from build123d import *

# Parameters (mm, degrees)
BASE_FLANGE3_DEPTH       = 425
SKETCH21_W               = 50
SKETCH21_H               = 5
BOSS_EXTRUDE2_DEPTH      = 50
CHAMFER1_SIZE            = 5
SKETCH26_R               = 9
CUT_EXTRUDE1_DEPTH       = 50
CHAMFER1_OF_MIRROR1_SIZE = 5


# Sheet-metal steps are written as plain solids
with BuildPart() as part:
    # Sketch1 → Base-Flange3 (new, symmetric)
    with BuildSketch(Plane.XY):
        with BuildLine():
            Line((63.8, 0), (63.8, 27.625))
            ThreePointArc((63.8, 27.625), (65.901508845, 32.698491155), (70.975, 34.8))
            Line((70.975, 34.8), (132.825, 34.8))
            ThreePointArc((132.825, 34.8), (137.898491155, 32.698491155), (140, 27.625))
            Line((140, 27.625), (140, 0))
            Line((140, 0), (136.825, 0))
            Line((136.825, 0), (136.825, 27.625))
            ThreePointArc((136.825, 27.625), (135.653427125, 30.453427125), (132.825, 31.625))
            Line((132.825, 31.625), (70.975, 31.625))
            ThreePointArc((70.975, 31.625), (68.146572875, 30.453427125), (66.975, 27.625))
            Line((66.975, 27.625), (66.975, 0))
            Line((66.975, 0), (63.8, 0))
        make_face()
    extrude(amount=BASE_FLANGE3_DEPTH, both=True)

    # Sketch21 → Boss-Extrude2 (add)
    with BuildSketch(Plane(origin=(140, 0, 0), x_dir=(0, 0, -1), z_dir=(1, 0, 0))):
        with Locations((-225, 2.5)):
            Rectangle(SKETCH21_W, SKETCH21_H)
    boss_extrude2 = extrude(amount=BOSS_EXTRUDE2_DEPTH)

    # Chamfer1
    chamfer1_edges = [part.edges().sort_by_distance(p)[0] for p in [
        (190, 2.5, 250),
        (190, 2.5, 200),
    ]]
    chamfer(chamfer1_edges, length=CHAMFER1_SIZE)

    # Sketch26 → Cut-Extrude1 (cut)
    with BuildSketch(Plane(origin=(0, 5, 0), x_dir=(1, 0, 0), z_dir=(0, 1, 0))):
        with Locations(Location((165, -225, 0), (0, 0, 270))):
            Circle(SKETCH26_R)
    cut_extrude1 = extrude(amount=-CUT_EXTRUDE1_DEPTH, mode=Mode.SUBTRACT)

    # Mirror1: Boss-Extrude2, Cut-Extrude1 across plane
    add(boss_extrude2.mirror(Plane.XY))
    add(cut_extrude1.mirror(Plane.XY), mode=Mode.SUBTRACT)

    # Chamfer1 of Mirror1
    chamfer1_of_mirror1_edges = [part.edges().sort_by_distance(p)[0] for p in [
        (190, 2.5, -250),
        (190, 2.5, -200),
    ]]
    chamfer(chamfer1_of_mirror1_edges, length=CHAMFER1_OF_MIRROR1_SIZE)


solid = part.part
Work out the finished part from the listing and answer in its coordinate system (mm). A direction names the side the tool comes from. Give positions to 0.01 mm unless a question says otherwise; leave off trailing zeros. Order: outer loops, then holes, each group sorted by start corner. A loop starts at its lowest first (then second) coordinate and runs counter-clockwise, first axis right, second up. Notation, with made-up numbers: (66.25, 66) - (78.25, 66) arc R19 ccw to (78.25, 84) - close; hole circle Ø8 at (67, 29.25). An arc over 180 degrees is marked (long way). Answer as CSV lines item,"result". Start each with the question number.
Q1. Find the intervals of material crossed by L1, parallel to X at y = 2.05, z = 225 (3 decimals); L2, parallel to X at y = 13, z = -217 (3 decimals); L3, parallel to Y at x = 83.5, z = 259.5 (3 decimals), in increasing order. Write a range as [from, to].
Q2. The part is cut by section B-B (z = -225). Write down the section's boundary in (x, y) (3 decimals).
Q3. The part is cut by section A-A (y = 21). Write down the section's boundary in (x, z) (3 decimals).
Q4. The part is cut by section D-D (z = 364.5). Write down the section's boundary in (x, y) (3 decimals), then the cut area to 3 significant figures.
Q5. For faces 4 (the face through (66.975, 14, 6)), 5 (the face through (165, 5, -214)), 6 (the face through (138, 0, -61)), determine the directions among +Z, -Z, +X, -X, +Y, -Y from which every point of the face is accessible in a straight line to the end or side of a thin tool.
Q6. Given pin 1 Ø18.5 at (x, z) = (117.5, 83.5) entering from -Y (3 decimals); pin 2 Ø14 at (y, z) = (20.5, -30.5) entering from +X; pin 3 Ø8 at (x, y) = (169, 7.5) entering from +Z, each flat-ended and moving along its own axis, determine where each tip first touches the part or whether it passes through.
Q7. The part is cut by section C-C (x = 165). Write down the section's boundary in (y, z).
Q8. The mould has two halves that part along Z. Classify faces 1 (the face through (102, 32, 425)), 2 (the face through (171.083, 2.535, -218.367)), 3 (the face through (102, 31.625, 6)): +Z half, -Z half, draft (parallel to the pull), parting line (faces both ways), or undercut.
Check result:
1,L1,"x = [63.8, 66.975], [136.825, 156], [174, 190]"
1,L2,"x = [63.8, 66.975], [136.825, 140]"
1,L3,"y = [31.625, 34.8]"
2,outline,"(63.8, 0) - (66.975, 0) - (66.975, 27.625) arc R4 cw to (70.975, 31.625) - (132.825, 31.625) arc R4 cw to (136.825, 27.625) - (136.825, 0) - (156, 0) - (156, 5) - (140, 5) - (140, 27.625) arc R7.175 ccw to (132.825, 34.8) - (70.975, 34.8) arc R7.175 ccw to (63.8, 27.625) - close; (174, 0) - (190, 0) - (190, 5) - (174, 5) - close"
3,outline,"(63.8, -425) - (66.975, -425) - (66.975, 425) - (63.8, 425) - close; (136.825, -425) - (140, -425) - (140, 425) - (136.825, 425) - close"
4,outline,"(63.8, 0) - (66.975, 0) - (66.975, 27.625) arc R4 cw to (70.975, 31.625) - (132.825, 31.625) arc R4 cw to (136.825, 27.625) - (136.825, 0) - (140, 0) - (140, 27.625) arc R7.175 ccw to (132.825, 34.8) - (70.975, 34.8) arc R7.175 ccw to (63.8, 27.625) - close"
4,area,"428 mm²"
5,face 4,"+Z, -Z, -Y"
5,face 5,"+Z, -Z, +X, +Y"
5,face 6,"+Z, -Z, +X, -X, -Y"
6,pin 1,"stops at y = 31.625"
6,pin 2,"stops at x = 140"
6,pin 3,"stops at z = 250"
7,outline,"(0, -250) - (5, -250) - (5, -234) - (0, -234) - close; (0, -216) - (5, -216) - (5, -200) - (0, -200) - close; (0, 200) - (5, 200) - (5, 216) - (0, 216) - close; (0, 234) - (5, 234) - (5, 250) - (0, 250) - close"
8,face 1,"+Z half"
8,face 2,"undercut"
8,face 3,"draft"
